from build123d import *

# Parameters (mm, degrees)
SKETCH_1_R          = 1.5
EXTRUDE_1_DEPTH     = 6
EXTRUDE_2_DEPTH     = 10
CUT_EXTRUDE_START   = -5
SKETCH_3_R          = 1.5
CUT_EXTRUDE_1_DEPTH = 5


with BuildPart() as part:
    # 草图1 → 凸台-拉伸1 (new body)
    with BuildSketch(Plane(origin=(0, 0, 0), x_dir=(1, 0, 0), z_dir=(0, 1, 0))):
        with Locations(Location((0, 0, 0), (0, 0, 270))):
            Circle(SKETCH_1_R)
    extrude(amount=EXTRUDE_1_DEPTH)

    # 草图2 → 凸台-拉伸2 (add)
    with BuildSketch(Plane(origin=(0, 6, 0), x_dir=(1, 0, 0), z_dir=(0, 1, 0))):
        Polygon((2.495784313, -1.136615149), (2.23222975, 1.593105043), (-0.263554563, 2.729720192), (-2.495784313, 1.136615149), (-2.23222975, -1.593105043), (0.263554563, -2.729720192), align=None)
    extrude(amount=EXTRUDE_2_DEPTH)

    # 草图3 → 切除-拉伸1 (cut)
    with BuildSketch(Plane(origin=(0, 16, 0), x_dir=(1, 0, 0), z_dir=(0, 1, 0)).offset(CUT_EXTRUDE_START)):
        with Locations(Location((0, 0, 0), (0, 0, 270))):
            Circle(SKETCH_3_R)
    extrude(amount=CUT_EXTRUDE_1_DEPTH, mode=Mode.SUBTRACT)


solid = part.part
Geometry: final body of the model. Coordinates: model frame, mm. A direction names the side the tool comes from. Give positions to 0.01 mm unless a question says otherwise; leave off trailing zeros. Write each loop counter-clockwise with the first axis right and the second up, starting at its lowest first coordinate (ties: lowest second). Pieces come first, ordered by that corner, then holes. Notation, with made-up numbers: (62.25, 4) - (86.25, 4) arc R20 ccw to (86.25, 36) - close; hole circle Ø7 at (-3, 36). An arc over 180 degrees is marked (long way). Return JSON: item names as keys, results as strings. Group by question number.
1) Section D-D on y = 9.5. Return the cut outline in (x, z).
2) First-contact query: P1, Ø1, axis at x = -1.5, y = 12.5, coming from the +Z side; P2, Ø1.5, axis at x = 2, y = 7.5, coming from the +Z side. Flat tips, straight axial feed; report the tip coordinate or a pass-through.
3) Line query: line 1 (Y direction, x = -0.3, z = -1.15); line 2 (Y direction, x = 2.2, z = -0.7); line 3 (X direction, y = 12.9, z = 0). Output: solid intervals per line, ascending.
4) Section A-A on y = 14.5. Return the cut outline in (x, z), plus the area to 3 significant figures.
5) Section B-B on z = 0. Return the cut outline in (x, y).
6) Section C-C on x = -0.8. Return the cut outline in (y, z), plus the area to 3 significant figures.
7) Set-up query: faces 1 (the flat face through (1.002, 10.93, -2.153)), 2 (the flat face through (1.1, 6, -1.3)), 3 (the cylindrical face through (0.45, 13.46, 1.43)). Return all of +Z, -Z, +X, -X, +Y, -Y with unobstructed straight access to the full face (end or side cutting, diameter ignored); none if empty.
8) Mould query, pull axis Z, two halves, no side actions, for faces 4 (the flat face through (-1.364, 10.93, -1.944)), 5 (the flat face through (1.364, 10.93, 1.944)), 6 (the flat face through (0, 11, 0)). Classes: released by +Z, released by -Z, zero draft, split by the parting line, or undercut.
Filled in:
{
 "1": {"outline": "(-2.5, -1.14) - (-0.26, -2.73) - (2.23, -1.59) - (2.5, 1.14) - (0.26, 2.73) - (-2.23, 1.59) - close"},
 "2": {"P1": "stops at z = 2.15", "P2": "stops at z = 2.03"},
 "3": {"line 1": "y = 0 to 11", "line 2": "y = 6 to 16", "line 3": "x = -2.39 to -1.5, 1.5 to 2.39"},
 "4": {"outline": "(-2.5, -1.14) - (-0.26, -2.73) - (2.23, -1.59) - (2.5, 1.14) - (0.26, 2.73) - (-2.23, 1.59) - close; hole circle Ø3 at (0, 0)", "area": "12.5 mm^2"},
 "5": {"outline": "(-2.39, 6) - (-1.5, 6) - (-1.5, 0) - (1.5, 0) - (1.5, 6) - (2.39, 6) - (2.39, 16) - (1.5, 16) - (1.5, 11) - (-1.5, 11) - (-1.5, 16) - (-2.39, 16) - close"},
 "6": {"outline": "(0, -1.27) - (6, -1.27) - (6, -2.35) - (16, -2.35) - (16, -1.27) - (11, -1.27) - (11, 1.27) - (16, 1.27) - (16, 2.25) - (6, 2.25) - (6, 1.27) - (0, 1.27) - close", "area": "48.5 mm^2"},
 "7": {"face 1": "-Z, +X, +Y, -Y", "face 2": "-Y", "face 3": "+Y"},
 "8": {"face 4": "released by -Z", "face 5": "released by +Z", "face 6": "undercut"}
}
